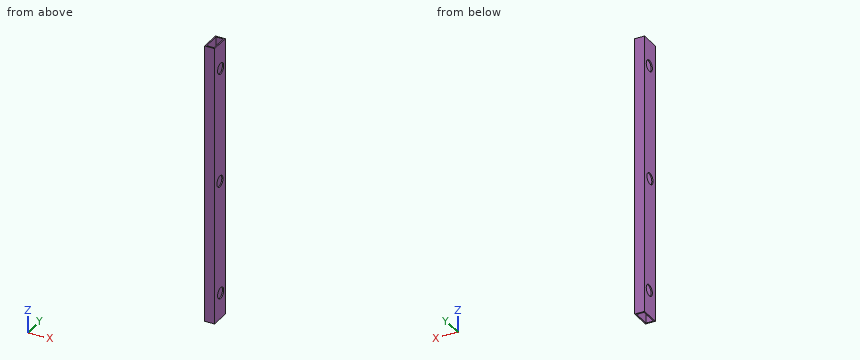
from build123d import *

# Parameters (mm, degrees)
SKETCH1_W           = 25.4
SKETCH1_H           = 50.8
SKETCH1_W_2         = 19.05
SKETCH1_H_2         = 44.45
BOSS_EXTRUDE1_DEPTH = 355.6
SKETCH2_R           = 14.2875
CUT_EXTRUDE1_DEPTH  = 446.225122831


with BuildPart() as part:
    # Sketch1 → Boss-Extrude1 (new body)
    with BuildSketch(Plane.XY):
        with Locations((254, 0)):
            Rectangle(SKETCH1_W, SKETCH1_H)
        with Locations((254, 0)):
            Rectangle(SKETCH1_W_2, SKETCH1_H_2, mode=Mode.SUBTRACT)
    boss_extrude1 = extrude(amount=BOSS_EXTRUDE1_DEPTH)

    # Mirror1: Boss-Extrude1 across plane
    add(boss_extrude1.mirror(Plane.XY))

    # Sketch2 → Cut-Extrude1 (cut, through all)
    with BuildSketch(Plane(origin=(0, 0, 0), x_dir=(0, 0, -1), z_dir=(1, 0, 0))):
        with Locations((290.007440579, 3.175)):
            Circle(SKETCH2_R)
        Circle(SKETCH2_R)
        with Locations((-290.007440579, 3.175)):
            Circle(SKETCH2_R)
    extrude(amount=CUT_EXTRUDE1_DEPTH, mode=Mode.SUBTRACT)


solid = part.part
Can you work these out from the model? Positions are in its coordinate system, mm. Round coordinates to 2 decimals unless told otherwise and drop trailing zeros. Write each loop counter-clockwise with the first axis right and the second up, starting at its lowest first coordinate (ties: lowest second). Pieces come first, ordered by that corner, then holes. Notation, with made-up numbers: (87, -11) -> (114, -11) arc R26 cw to (114, 27) -> close; hole circle Ø10 at (15.5, 66.5). An arc over 180 degrees is marked (long way). Use one line per item in the form item = value. Start each with the question number.
Q1. I'm going to push a flat-ended pin straight in: P1, Ø23, axis at y = 3.18, z = -290.01, coming from the +X side. Where does the tip first touch, or does it pass through?
Q2. Imagine slicing it at B-B (x = 254.75). Please give me the cut outline in (y, z) (3 decimals).
Q3. If I drill on probe 1 along Y at (x, z) = (256.25, -141.5) (3 decimals); probe 2 along X at (y, z) = (-13, -9) (3 decimals); probe 3 along Y at (x, z) = (265.25, 0), over which ranges is the centre line in solid material (lowest first)? Write a range as [from, to].
Q4. Imagine slicing it at C-C (z = -204). Please give me the cut outline in (x, y) (3 decimals).
Q5. Imagine slicing it at A-A (z = 0). Please give me the cut outline in (x, y) (1 decimal), then the cut area to 3 significant figures.
Worked out:
q1.P1 = through
q2.outline = (-25.4, -355.6) -> (-22.225, -355.6) -> (-22.225, 355.6) -> (-25.4, 355.6) -> close; (22.225, -355.6) -> (25.4, -355.6) -> (25.4, 355.6) -> (22.225, 355.6) -> close
q3.probe_1 = [-25.4, -22.225], [22.225, 25.4]
q3.probe_2 = [241.3, 244.475], [263.525, 266.7]
q3.probe_3 = [-25.4, -14.29], [14.29, 25.4]
q4.outline = (241.3, -25.4) -> (266.7, -25.4) -> (266.7, 25.4) -> (241.3, 25.4) -> close; hole (244.475, -22.225) -> (263.525, -22.225) -> (263.525, 22.225) -> (244.475, 22.225) -> close
q5.outline = (241.3, -25.4) -> (266.7, -25.4) -> (266.7, -14.3) -> (263.5, -14.3) -> (263.5, -22.2) -> (244.5, -22.2) -> (244.5, -14.3) -> (241.3, -14.3) -> close; (241.3, 14.3) -> (244.5, 14.3) -> (244.5, 22.2) -> (263.5, 22.2) -> (263.5, 14.3) -> (266.7, 14.3) -> (266.7, 25.4) -> (241.3, 25.4) -> close
q5.area = 262 mm^2
